For this review, take the finished solid that the model builds, in its own axes (mm). A direction names the side the tool comes from. Coordinates: 2 decimals unless noted, no trailing zeros. Loops run counter-clockwise (first coordinate to the right, second up) from the corner with the lowest first, then second, coordinate; pieces in that order, holes last.
1. Clearance check with flat-ended pins moving along their axes: P1, Ø5, axis at x = -31.5, y = 17, coming from the +Z side; P2, Ø2.5, axis at x = 37, y = 34, coming from the +Z side; P3, Ø0.6, axis at x = -38, z = 9, coming from the +Y side. State where each tip first meets the part, or that it passes through.
2. To check wall thickness, follow probe 1 along X at (y, z) = (6, 1.5); probe 2 along X at (y, z) = (-11, 8.5); probe 3 along Y at (x, z) = (20, -5.5). State the ranges of each line that lie inside material, in increasing order.
3. Take a section at D-D, the plane x = -3.5. State the section outline as (y, z) points, then the cut area to 3 significant figures.
4. Take a section at B-B, the plane z = 6.25. State the section outline as (x, y) points.
5. Machinability: for faces 1 (the face through (0, -12, 5.25)), 2 (the face through (-25, 15, 2)), 3 (the face through (-21, 15, 1)), 4 (the face through (37, 29, 7.75)), which of the approach directions +Z, -Z, +X, -X, +Y, -Y give a long, thin tool a straight path to every point of the face, cutting with its end or side? Answer none if there is none.
6. Mouldability with a two-part tool opening along X and no side actions: class faces 5 (the face through (22, 29, 7.75)), 6 (the face through (1, -15, 1)) as pulls with the +X half, pulls with the -X half, needs draft (parallel to the pull), parting line crosses it, or undercut.
7. Take a section at C-C, the plane z = -1.75. State the section outline as (x, y) points, then the cut area to 3 significant figures.
8. Take a section at A-A, the plane y = -5. State the section outline as (x, z) points, then the cut area to 3 significant figures.
```python
from build123d import *

# Parameters (mm, degrees)
F1_DEPTH  = 40
F2_W      = 4
F2_H      = 0.5
F3_DEPTH  = 18
F5_W      = 1
F5_H      = 22
F6_DEPTH  = 0.5
F4_W      = 10
F4_H      = 6.25
F4_H_2    = 5.75
F7_DEPTH  = 15
F9_DEPTH  = 36.001
F10_DEPTH = 5.75
F11_DEPTH = 7
F12_DEPTH = 10
F14_DEPTH = 1.5


with BuildPart() as f1:
    # F0 (on Front) → F1 (new body)
    with BuildSketch(Plane.XZ):
        Polygon((-25, 2), (-35, 2), (-35, 7.75), (-39, 7.75), (-39, -7.75), (-35, -7.75), (-35, -2), (-25, -2), (-25, -7.75), (-21, -7.75), (-21, 7.75), (-25, 7.75), align=None)
    extrude(amount=-F1_DEPTH)

    # F2 (on face) → F3 (join)
    with BuildSketch(Plane.XZ):
        with Locations((-37, 8)):
            Rectangle(F2_W, F2_H)
        with Locations((-23, 8)):
            Rectangle(F2_W, F2_H)
    extrude(amount=-F3_DEPTH)

    # F5 (on face) → F6 (join)
    with BuildSketch(Plane.XY.offset(7.75)):
        with Locations((-35.5, 29)):
            Rectangle(F5_W, F5_H)
        with Locations((-24.5, 29)):
            Rectangle(F5_W, F5_H)
    extrude(amount=F6_DEPTH)

    # F4 (on face) → F7 (join)
    with BuildSketch(Plane.XZ):
        with Locations((-30, 5.125)):
            Rectangle(F4_W, F4_H)
        Polygon((-35, 8.25), (-39, 8.25), (-39, -7.75), (-35, -7.75), (-35, -2), (-25, -2), (-25, -7.75), (-21, -7.75), (-21, 8.25), (-25, 8.25), (-25, 2), (-35, 2), align=None)
        with Locations((-30, -4.875)):
            Rectangle(F4_W, F4_H_2)
        Polygon((-14, 8.25), (-21, 8.25), (-21, -7.75), (-13.5, -7.75), (0, -7.75), (0, 5.25), (-14, 5.25), align=None)
    extrude(amount=F7_DEPTH)

    # F8 (on face) → F9 (cut, through all)
    with BuildSketch(Plane(origin=(-36, 0, 0), x_dir=(0, -1, 0), z_dir=(-1, 0, 0))):
        Polygon((-40, 8.25), (-40, 7.75), (-18, 8), (-18, 8.25), align=None)
    extrude(amount=-F9_DEPTH, mode=Mode.SUBTRACT)

    # F10 (add, through all): a face of the model
    f10_faces = [f1.faces().sort_by_distance(p)[0] for p in [
        (-30, 20, -2),
    ]]
    extrude(f10_faces, amount=F10_DEPTH)

    # F11 (cut): a face of the model
    f11_faces = [f1.faces().sort_by_distance(p)[0] for p in [
        (-30, 20, 2),
    ]]
    extrude(f11_faces, amount=-F11_DEPTH, mode=Mode.SUBTRACT)

    # F12 (cut): faces of the model
    f12_faces = [f1.faces().sort_by_distance(p)[0] for p in [
        (-11, 0, -0.6785714286),
        (-30, 0, 1.625),
        (-11, 0, -0.6785714286),
    ]]
    extrude(f12_faces, amount=-F12_DEPTH, mode=Mode.SUBTRACT)

    # F13: F1 across plane


with BuildPart() as f1_1:
    add(f1.part)
    add(f1.part.mirror(Plane.YZ))

    # F14 (add): faces of the model
    f14_faces = [f1_1.faces().sort_by_distance(p)[0] for p in [
        (-21.4140048309, 4, 8.25),
        (21.4140048309, 4, 8.25),
    ]]
    extrude(f14_faces, amount=F14_DEPTH)


solid = f1_1.part
```
Results list:
1. P1: stops at z = -5
1. P2: stops at z = 7.83
1. P3: stops at y = 18
2. probe 1: x = -39 to -35, -25 to -21, 21 to 25, 35 to 39
2. probe 2: x = -39 to -14, 14 to 39
2. probe 3: y = -15 to -10
3. outline: (-15, -7.75) - (-10, -7.75) - (-10, 5.25) - (-15, 5.25) - close
3. area: 65.0 mm2
4. outline: (-39, -15) - (-14, -15) - (-14, -10) - (-21, -10) - (-21, 40) - (-25, 40) - (-25, -10) - (-35, -10) - (-35, 40) - (-39, 40) - close; (14, -15) - (39, -15) - (39, 40) - (35, 40) - (35, -10) - (25, -10) - (25, 40) - (21, 40) - (21, -10) - (14, -10) - close
5. face 1: +Z, +Y, -Y
5. face 2: +Z, +Y
5. face 3: +Z, -Z, +Y
5. face 4: +Z, +X, +Y
6. face 5: undercut
6. face 6: needs draft
7. outline: (-39, -15) - (39, -15) - (39, 40) - (35, 40) - (35, -10) - (25, -10) - (25, 40) - (21, 40) - (21, -10) - (-21, -10) - (-21, 40) - (-25, 40) - (-25, -10) - (-35, -10) - (-35, 40) - (-39, 40) - close
7. area: 1,190 mm2
8. outline: (-39, -7.75) - (-21, -7.75) - (-21, 9.75) - (-25, 9.75) - (-25, -5) - (-35, -5) - (-35, 9.75) - (-39, 9.75) - close; (21, -7.75) - (39, -7.75) - (39, 9.75) - (35, 9.75) - (35, -5) - (25, -5) - (25, 9.75) - (21, 9.75) - close
8. area: 335 mm2
